Can you work these out from the model? Positions are in its coordinate system, mm. A direction names the side the tool comes from. Round coordinates to 2 decimals unless told otherwise and drop trailing zeros. Order: outer loops, then holes, each group sorted by start corner. A loop starts at its lowest first (then second) coordinate and runs counter-clockwise, first axis right, second up.
from build123d import *

# Parameters (mm, degrees)
SKETCH_1_W     = 25
SKETCH_1_H     = 7.5
SKETCH_1_W_2   = 10
SKETCH_1_H_2   = 40
CHAMFER_1_SIZE = 10
CHAMFER_2_SIZE = 10
CHAMFER_3_SIZE = 3


with BuildPart() as part:
    # 草圖1 → 迴轉1 (revolve)
    with BuildSketch(Plane.XY, mode=Mode.PRIVATE) as revolve_1_sk:
        with Locations((12.5, 3.75)):
            Rectangle(SKETCH_1_W, SKETCH_1_H)
        with Locations((145, 20)):
            Rectangle(SKETCH_1_W_2, SKETCH_1_H_2)
        Polygon((25, 7.5), (25, 0), (140, 0), (140, 20), (25, 20), align=None)
    revolve(revolve_1_sk.sketch.rotate(Axis((25, 0, 0), (1, 0, 0)), 90), axis=Axis((25, 0, 0), (1, 0, 0)))

    # 倒角1
    chamfer_1_edges = [part.edges().sort_by_distance(p)[0] for p in [
        (150, 0, -40),
    ]]
    chamfer(chamfer_1_edges, length=CHAMFER_1_SIZE - 0.0001)  # a hair under: the kernel refuses the full size

    # 倒角2
    chamfer_2_edges = [part.edges().sort_by_distance(p)[0] for p in [
        (140, 0, -20),
    ]]
    chamfer(chamfer_2_edges, length=CHAMFER_2_SIZE)

    # 倒角3
    chamfer_3_edges = [part.edges().sort_by_distance(p)[0] for p in [
        (25, 0, -20),
    ]]
    chamfer(chamfer_3_edges, length=CHAMFER_3_SIZE)


solid = part.part
(1) I want a section at C-C, the plane x = 38.5. List the corners of the cut face in (y, z) for me, plus the area to 3 significant figures.
(2) On a 3-axis mill with a long thin cutter (end or side, diameter ignored), from which of +Z, -Z, +X, -X, +Y, -Y can I reach the whole of each face in a straight line? I mean faces 1 (the face through (78.29, -0.88, -19.98)), 2 (the face through (149.374, -9.199, 29.211)). Say none if no direction works.
(3) I'm going to push flat-ended pins straight in: pin 1 Ø12 at (x, z) = (73.5, 0) entering from -Y; pin 2 Ø2 at (x, z) = (28.5, -9) entering from +Y; pin 3 Ø4 at (y, z) = (21.5, -30.5) entering from +X. Where does each tip first touch, or does it pass through?
(4) Please list where these lines run through material, in increasing order: probe 1 along Z at (x, y) = (113.5, 17.5); probe 2 along Y at (x, z) = (75, -13); probe 3 along Z at (x, y) = (113, -18.5).
Ans:
1. outline: circle Ø40 at (0, 0)
1. area: 1,260 mm2
2. face 1: -X
2. face 2: +X
3. pin 1: stops at y = -20
3. pin 2: stops at y = 18.33
3. pin 3: stops at x = 144.68
4. probe 1: z = -9.68 to 9.68
4. probe 2: y = -15.2 to 15.2
4. probe 3: z = -7.6 to 7.6
